Can you work these out from the model? Positions are in its coordinate system, mm. A direction names the side the tool comes from. Give positions to 0.01 mm unless a question says otherwise; leave off trailing zeros. Loops run counter-clockwise (first coordinate to the right, second up) from the corner with the lowest first, then second, coordinate; pieces in that order, holes last. Notation, with made-up numbers: (62, -5.5) - (80, -5.5) arc R31 ccw to (80, 28.5) - close; hole circle Ø5 at (69, -14). An arc over 180 degrees is marked (long way). Write item = value, one per line.
from build123d import *

# Parameters (mm, degrees)
SKETCH113_R     = 75.75
PAD051_DEPTH    = 50
THICKNESS001_T  = -2
SKETCH114_R     = 8
POCKET112_DEPTH = 2.001


with BuildPart() as part:
    # Sketch113 → Pad051 (new body)
    with BuildSketch(Plane.XY.offset(-30)):
        Circle(SKETCH113_R)
    extrude(amount=-PAD051_DEPTH)

    # Thickness001
    thickness001_openings = [part.faces().sort_by_distance(p)[0] for p in [
        (0, 0, -30),
    ]]
    offset(amount=THICKNESS001_T, openings=thickness001_openings)

    # Sketch114 (on Face5 of Thickness001) → Pocket112 (cut, through all)
    with BuildSketch(Plane.XY.offset(-78)):
        Circle(SKETCH114_R)
    extrude(amount=-POCKET112_DEPTH, mode=Mode.SUBTRACT)


with BuildPart() as part_1:
    # Body007 placement: moved
    add(part.part.moved(Location((0, 0, 5.75))))


solid = part_1.part
Q1. Imagine slicing it at A-A, the plane x = 0. Write out the boundary of the cut face in (y, z), then the cut area to 3 significant figures.
Output:
outline = (-75.75, -74.25) - (-8, -74.25) - (-8, -72.25) - (-73.75, -72.25) - (-73.75, -24.25) - (-75.75, -24.25) - close; (8, -74.25) - (75.75, -74.25) - (75.75, -24.25) - (73.75, -24.25) - (73.75, -72.25) - (8, -72.25) - close
area = 463 mm2
Q2. Which directions (+Z, -Z, +X, -X, +Y, -Y) give clear straight access to the entire face, cutting with the end or side of a thin tool? Please do faces 4 (the cylindrical face through (-15.988, -71.996, -47.914)), 5 (the cylindrical face through (-1.73, -7.81, -73.24)).
Output:
face_4 = +Z
face_5 = +Z, -Z
Q3. Imagine slicing it at C-C, the plane z = -37.5. Write out the boundary of the cut face in (x, y), then the cut area to 3 significant figures.
Output:
outline = circle Ø151.5 at (0, 0); hole circle Ø147.5 at (0, 0)
area = 939 mm2
Q4. Imagine slicing it at D-D, the plane y = -56. Write out the boundary of the cut face in (x, z).
Output:
outline = (-51.01, -74.25) - (51.01, -74.25) - (51.01, -24.25) - (47.99, -24.25) - (47.99, -72.25) - (-47.99, -72.25) - (-47.99, -24.25) - (-51.01, -24.25) - close
Q5. For pin 1 (1 mm diameter, centred on x = -28.5, z = -48.5, fed in from -Y); pin 2 (4 mm diameter, centred on x = 11.5, z = -66, fed in from +Y); pin 3 (6 mm diameter, centred on x = 41, z = -65, fed in from +Y); pin 4 (1.5 mm diameter, centred on y = -0.5, z = -57.5, fed in from +X), each with a flat end and sliding along its axis, tell me the tip position at first contact or that it passes through.
Output:
pin_1 = -70.39
pin_2 = 75.15
pin_3 = 65.53
pin_4 = 75.75
Q6. We'd pull the mould along X, two halves only. Please class faces 1 (the flat face through (16, -73, -24.25)), 2 (the cylindrical face through (-75.677, 3.331, -48.9)), 3 (the flat face through (-1, -15, -72.25)): released by +X, released by -X, zero draft, split by the parting line, or undercut.
Output:
face_1 = zero draft
face_2 = split by the parting line
face_3 = undercut
Q7. I need wall thicknesses on L1, parallel to Y at x = 0, z = -52; L2, parallel to Y at x = 0, z = -73.6; L3, parallel to Z at x = -61, y = -34. Which ranges of each line are inside material? Lowest first, please.
Output:
L1 = -75.75 to -73.75, 73.75 to 75.75
L2 = -75.75 to -8, 8 to 75.75
L3 = -74.25 to -72.25
